Design review of the part built by this model. Coordinates are the model's own, in mm. A direction names the side the tool comes from. Coordinates: 2 decimals unless noted, no trailing zeros. Write each loop counter-clockwise with the first axis right and the second up, starting at its lowest first coordinate (ties: lowest second). Pieces come first, ordered by that corner, then holes. Notation, with made-up numbers: (-7, 72) - (4, 72) arc R3 cw to (4, 76) - close; hole circle Ø9 at (73.5, -9). An arc over 180 degrees is marked (long way). Answer as a JSON object with one key per item and string values.
```python
from build123d import *

# Parameters (mm, degrees)
BOSS_EXTRUDE1_DEPTH       = 38.1
SKETCH3_W                 = 50.8
SKETCH3_H                 = 32.3088
BOSS_EXTRUDE2_DEPTH       = 2.54
SHELL2_T                  = -2.54
SKETCH5_R                 = 2.54
BOSS_EXTRUDE3_DEPTH       = 2.54
F_4_40_TAPPED_HOLE1_D     = 2.2606
F_4_40_TAPPED_HOLE1_DEPTH = 98.926014438
F_4_40_TAPPED_HOLE1_TIP   = 0.679152758
CUT_EXTRUDE1_DEPTH        = 2.54
CIRPATTERN1_COUNT         = 4


with BuildPart() as part:
    # Sketch1 → Boss-Extrude1 (new body)
    with BuildSketch(Plane(origin=(0, 0, 0), x_dir=(1, 0, 0), z_dir=(0, 1, 0))):
        Polygon((0, 0), (57.15, 0), (57.15, 41.777014438), (120.65, 41.777014438), (120.65, 98.927014438), (57.15, 98.927014438), (0, 38.1), align=None)
    extrude(amount=BOSS_EXTRUDE1_DEPTH)

    # Sketch3 → Boss-Extrude2 (add)
    with BuildSketch(Plane.XY):
        with Locations((28.575, 19.05)):
            Rectangle(SKETCH3_W, SKETCH3_H)
    extrude(amount=BOSS_EXTRUDE2_DEPTH)

    # Shell2
    shell2_openings = [part.faces().sort_by_distance(p)[0] for p in [
        (28.575, 19.05, 2.54),
    ]]
    offset(amount=SHELL2_T, openings=shell2_openings, kind=Kind.INTERSECTION)

    # Sketch5 → Boss-Extrude3 (add)
    with BuildSketch(Plane.XY.offset(2.54)):
        with Locations((3.175, 19.05)):
            Circle(SKETCH5_R)
        with Locations((53.975, 19.05)):
            Circle(SKETCH5_R)
    extrude(amount=-BOSS_EXTRUDE3_DEPTH)

    # #4-40 Tapped Hole1
    with Locations(Plane(origin=(53.975, 19.05, 2.54), x_dir=(1, 0, 0), z_dir=(0, 0, 1))):
        with Locations((0, 0), (-50.8, 0)):
            Hole(F_4_40_TAPPED_HOLE1_D / 2, depth=F_4_40_TAPPED_HOLE1_DEPTH)
            with Locations((0, 0, -(F_4_40_TAPPED_HOLE1_DEPTH + F_4_40_TAPPED_HOLE1_TIP / 2))):  # 118° drill point
                Cone(0, F_4_40_TAPPED_HOLE1_D / 2, F_4_40_TAPPED_HOLE1_TIP, mode=Mode.SUBTRACT)

    # single button hole → Cut-Extrude1 (cut)
    with BuildSketch(Plane(origin=(0, 0, -98.927014438), x_dir=(-1, 0, 0), z_dir=(0, 0, -1))):
        with BuildLine():
            Line((-93.345, 10.668), (-97.155, 10.668))
            ThreePointArc((-97.155, 10.668), (-99.187, 12.7), (-97.155, 14.732))
            Line((-97.155, 14.732), (-93.345, 14.732))
            ThreePointArc((-93.345, 14.732), (-91.313, 12.7), (-93.345, 10.668))
        make_face()
    cut_extrude1 = extrude(amount=-CUT_EXTRUDE1_DEPTH, mode=Mode.SUBTRACT)

    # CirPattern1: Cut-Extrude1 ×4 about axis
    cirpattern1_axis = Axis((95.25, 19.05, 0), (0, 0, 1))
    for i in range(1, CIRPATTERN1_COUNT):
        add(cut_extrude1.rotate(cirpattern1_axis, i * 360 / CIRPATTERN1_COUNT), mode=Mode.SUBTRACT)


solid = part.part
```
(1) Take a section at A-A, the plane y = 25.4. Write out the cut boundary in (x, z) (3 decimals), and give its area (3 significant figures).
Solved:
{"outline": "(0, -38.1) - (57.15, -98.927) - (91.313, -98.927) - (91.313, -96.387) - (58.249, -96.387) - (2.54, -37.094) - (2.54, -2.54) - (5.715, -2.54) - (5.715, 2.54) - (3.175, 2.54) - (3.175, 0) - (0, 0) - close; (51.435, -2.54) - (54.61, -2.54) - (54.61, -44.317) - (118.11, -44.317) - (118.11, -96.387) - (99.187, -96.387) - (99.187, -98.927) - (120.65, -98.927) - (120.65, -41.777) - (57.15, -41.777) - (57.15, 0) - (53.975, 0) - (53.975, 2.54) - (51.435, 2.54) - close", "area": "880 mm^2"}
(2) Take a section at B-B, the plane z = -30. Write out the cut boundary in (x, y) (3 decimals), and give its area (3 significant figures).
Solved:
{"outline": "(0, 0) - (57.15, 0) - (57.15, 38.1) - (0, 38.1) - close; hole (2.54, 2.54) - (54.61, 2.54) - (54.61, 18.115) arc R1.13 ccw to (54.61, 19.985) - (54.61, 35.56) - (2.54, 35.56) - (2.54, 19.985) arc R1.13 ccw to (2.54, 18.115) - close", "area": "457 mm^2"}
(3) The part is to be moulded in two halves that separate along X. For faces 1 (the face through (28, 35.204, 1)), 2 (the face through (57.15, 19, -21)), 3 (the face through (60, 2.54, -50)), say which applies: pulls with the +X half, pulls with the -X half, needs draft (parallel to the pull), parting line crosses it, or undercut.
Solved:
{"face 1": "needs draft", "face 2": "pulls with the +X half", "face 3": "undercut"}
(4) For pin 1 (16.5 mm diameter, centred on x = 26, y = 20.5, fed in from -Z); pin 2 (4 mm diameter, centred on y = 23, z = 0.5, fed in from +X); pin 3 (6 mm diameter, centred on y = 6, z = -82, fed in from -X); pin 4 (1.4 mm diameter, centred on x = 53.975, y = 19.05, fed in from -Z), all flat-tipped, find the tip position at first contact; note any pin that passes through.
Solved:
{"pin 1": "stops at z = -74.55", "pin 2": "stops at x = 57.15", "pin 3": "stops at x = 38.43", "pin 4": "passes through"}
(5) Take a section at D-D, the plane y = 8.5. Write out the cut boundary in (x, z) (3 decimals).
Solved:
{"outline": "(0, -38.1) - (57.15, -98.927) - (120.65, -98.927) - (120.65, -41.777) - (57.15, -41.777) - (57.15, 0) - (53.975, 0) - (53.975, 2.54) - (51.435, 2.54) - (51.435, -2.54) - (54.61, -2.54) - (54.61, -44.317) - (118.11, -44.317) - (118.11, -96.387) - (58.249, -96.387) - (2.54, -37.094) - (2.54, -2.54) - (5.715, -2.54) - (5.715, 2.54) - (3.175, 2.54) - (3.175, 0) - (0, 0) - close"}
(6) Tool access review of faces 4 (the face through (28, 2.896, 1)), 5 (the face through (82, 19, -96.387)), 6 (the face through (28, 32.664, 0)), 7 (the face through (3.175, 28, 1)), 8 (the face through (91.313, 25.445, -97.675)): name each direction out of +Z, -Z, +X, -X, +Y, -Y from which nothing blocks a thin tool from reaching the whole face with its end or side.
Solved:
{"face 4": "+Z, +X, -X, -Y", "face 5": "none", "face 6": "+Z", "face 7": "+Z, -X, +Y", "face 8": "-Z"}
(7) To check wall thickness, follow line 1 (Y direction, x = 26, z = -16.5); line 2 (X direction, y = 8.5, z = -11.5); line 3 (X direction, y = 19.05, z = -11.5). State the ranges of each line that lie inside material, in increasing order. Write a range as from..to.
Solved:
{"line 1": "y = 0..2.54, 35.56..38.1", "line 2": "x = 0..2.54, 54.61..57.15", "line 3": "x = 0..2.04, 55.11..57.15"}
(8) Take a section at C-C, the plane x = 101.6. Write out the cut boundary in (y, z), and give its area (3 significant figures).
Solved:
{"outline": "(0, -98.93) - (15.11, -98.93) - (15.11, -96.39) - (2.54, -96.39) - (2.54, -44.32) - (35.56, -44.32) - (35.56, -96.39) - (22.99, -96.39) - (22.99, -98.93) - (38.1, -98.93) - (38.1, -41.78) - (0, -41.78) - close", "area": "438 mm^2"}
